from build123d import *

# Parameters (mm, degrees)
SKETCH_1_R          = 8
SKETCH_1_W          = 38.5
SKETCH_1_H          = 12.4
SKETCH_1_W_2        = 22.5
SKETCH_1_H_2        = 8
EXTRUDE_1_DEPTH     = 35.25
CUT_EXTRUDE_1_DEPTH = 55.5
SKETCH_3_W          = 1.8
SKETCH_3_H          = 5.4
SKETCH_3_W_2        = 10
SKETCH_3_H_2        = 3
CUT_EXTRUDE_2_DEPTH = 2
SKETCH_4_W          = 1.8
SKETCH_4_H          = 5.4
CUT_EXTRUDE_3_DEPTH = 4.5


with BuildPart() as part:
    # 草图1 → 凸台-拉伸1 (new, symmetric)
    with BuildSketch(Plane.XY):
        with Locations((-11.25, 2.2)):
            Circle(SKETCH_1_R)
        with Locations((11.25, 2.2)):
            Circle(SKETCH_1_R)
        with Locations((0, -4)):
            Rectangle(SKETCH_1_W, SKETCH_1_H)
        with Locations((0, 6.2)):
            Rectangle(SKETCH_1_W_2, SKETCH_1_H_2)
    extrude(amount=EXTRUDE_1_DEPTH, both=True)

    # 草图2 → 切除-拉伸1 (cut)
    with BuildSketch(Plane(origin=(0, 0, -35.25), x_dir=(-1, 0, 0), z_dir=(0, 0, -1))):
        Polygon((-2.8, 10.2), (2.8, 10.2), (1.7, 7.5), (-1.7, 7.5), align=None)
    cut_extrude_1 = extrude(amount=-CUT_EXTRUDE_1_DEPTH, mode=Mode.SUBTRACT)

    # 草图3 → 切除-拉伸2 (cut)
    with BuildSketch(Plane.ZY.offset(19.25)):
        with Locations((-34.35, -7.5)):
            Rectangle(SKETCH_3_W, SKETCH_3_H)
        Polygon((-25.05, -10.2), (-21.15, -6.017762031), (-6.45, -6.017762031), (-6.45, -8.317762031), (-9.45, -8.317762031), (-12.95, -8.7), (-12.95, -10.2), align=None)
        with Locations((2.55, -8.7)):
            Rectangle(SKETCH_3_W_2, SKETCH_3_H_2)
        Polygon((12.95, -10.2), (16.85, -6.017762031), (31.55, -6.017762031), (31.55, -8.317762031), (28.55, -8.317762031), (25.05, -8.7), (25.05, -10.2), align=None)
    cut_extrude_2 = extrude(amount=-CUT_EXTRUDE_2_DEPTH, mode=Mode.SUBTRACT)

    # 草图4 → 切除-拉伸3 (cut)
    with BuildSketch(Plane.ZY.offset(17.25)):
        with Locations((-34.35, -7.5)):
            Rectangle(SKETCH_4_W, SKETCH_4_H)
    cut_extrude_3 = extrude(amount=-CUT_EXTRUDE_3_DEPTH, mode=Mode.SUBTRACT)

    # 镜向1: 切除-拉伸1, 切除-拉伸2, 切除-拉伸3 across plane
    add(cut_extrude_1.mirror(Plane(origin=(0, 0, 0), x_dir=(0, 0, 1), z_dir=(1, 0, 0))), mode=Mode.SUBTRACT)
    add(cut_extrude_2.mirror(Plane(origin=(0, 0, 0), x_dir=(0, 0, 1), z_dir=(1, 0, 0))), mode=Mode.SUBTRACT)
    add(cut_extrude_3.mirror(Plane(origin=(0, 0, 0), x_dir=(0, 0, 1), z_dir=(1, 0, 0))), mode=Mode.SUBTRACT)


solid = part.part
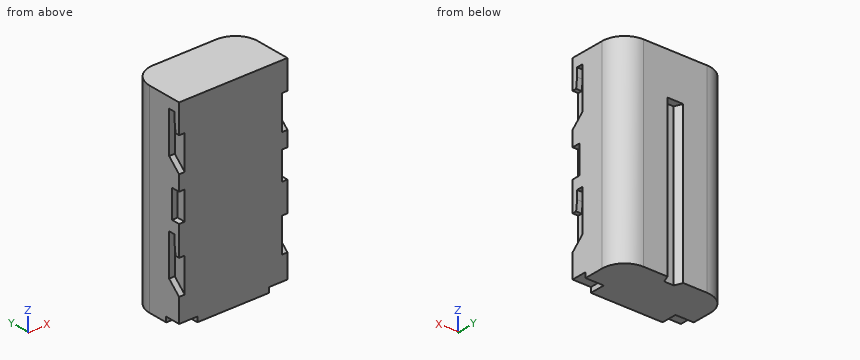
Build history of the part. All positions in model axes, mm. Round coordinates to 2 decimals unless told otherwise and drop trailing zeros. Loops run counter-clockwise (first coordinate to the right, second up) from the corner with the lowest first, then second, coordinate; pieces in that order, holes last. Notation, with made-up numbers: (-9, 5) -> (50, 5) arc R16 ccw to (50, 20) -> close; hole circle Ø2 at (85.5, 31.25). An arc over 180 degrees is marked (long way). Answer in a Markdown table with one row per item.
Item 1: Pin check, flat tips, straight feed: pin 1 (1 mm diameter, centred on x = -18, y = -7, fed in from -Z); pin 2 (0.6 mm diameter, centred on x = 18.5, z = 4, fed in from -Y); pin 3 (3 mm diameter, centred on x = 2, z = -22.5, fed in from +Y); pin 4 (1.3 mm diameter, centred on x = -1, y = 9, fed in from -Z). Stop position of each tip, or through.
Answers below:
| item | result |
|---|---|
| pin 1 | stops at z = -33.45 |
| pin 2 | stops at y = -7.2 |
| pin 3 | stops at y = 10.2 |
| pin 4 | stops at z = 20.25 |
Item 2: Drill centre lines: L1, parallel to Y at x = -0.5, z = 16; L2, parallel to X at y = 8.75, z = 17; L3, parallel to X at y = 8, z = -1. Where is each one in solid material? Low to high. Write a range as [from, to].
Answers below:
| item | result |
|---|---|
| L1 | y = [-10.2, 7.5] |
| L2 | x = [-15.84, -2.21], [2.21, 15.84] |
| L3 | x = [-16.76, -1.9], [1.9, 16.76] |
Item 3: Saw through at A-A (z = 2). Write the cut outline in (x, y).
Answers below:
| item | result |
|---|---|
| outline | (-19.25, -7.2) -> (-17.25, -7.2) -> (-17.25, -10.2) -> (17.25, -10.2) -> (17.25, -7.2) -> (19.25, -7.2) -> (19.25, 2.2) arc R8 ccw to (11.25, 10.2) -> (2.8, 10.2) -> (1.7, 7.5) -> (-1.7, 7.5) -> (-2.8, 10.2) -> (-11.25, 10.2) arc R8 ccw to (-19.25, 2.2) -> close |
Item 4: Saw through at C-C (z = 18). Write the cut outline in (x, y), and give its area (3 significant figures).
Answers below:
| item | result |
|---|---|
| outline | (-19.25, -6.02) -> (-17.25, -6.02) -> (-17.25, -10.2) -> (17.25, -10.2) -> (17.25, -6.02) -> (19.25, -6.02) -> (19.25, 2.2) arc R8 ccw to (11.25, 10.2) -> (2.8, 10.2) -> (1.7, 7.5) -> (-1.7, 7.5) -> (-2.8, 10.2) -> (-11.25, 10.2) arc R8 ccw to (-19.25, 2.2) -> close |
| area | 729 mm² |
Item 5: Saw through at B-B (x = 0.5). Write the cut outline in (y, z), and give its area (3 significant figures).
Answers below:
| item | result |
|---|---|
| outline | (-10.2, -35.25) -> (7.5, -35.25) -> (7.5, 20.25) -> (10.2, 20.25) -> (10.2, 35.25) -> (-10.2, 35.25) -> close |
| area | 1,290 mm² |
Item 6: Saw through at D-D (y = 5.25). Write the cut outline in (x, z), and give its area (3 significant figures).
Answers below:
| item | result |
|---|---|
| outline | (-18.65, -35.25) -> (18.65, -35.25) -> (18.65, 35.25) -> (-18.65, 35.25) -> close |
| area | 2,630 mm² |
